Verification items for the finished model (mm, model axes). Round coordinates to 2 decimals unless told otherwise and drop trailing zeros. Write each loop counter-clockwise with the first axis right and the second up, starting at its lowest first coordinate (ties: lowest second). Pieces come first, ordered by that corner, then holes. Notation, with made-up numbers: (45, -3) -> (78, -3) arc R29 cw to (78, 36) -> close; hole circle Ø1 at (-6, 58). An arc over 180 degrees is marked (long way). Use CSV: the item, a comma, the result in double quotes.
```python
from build123d import *

# Parameters (mm, degrees)
BOSS_EXTRUDE1_DEPTH = 119.85625
SKETCH2_R           = 2.032
CUT_EXTRUDE1_DEPTH  = 136.095780221
SKETCH3_R           = 2.032
CUT_EXTRUDE2_DEPTH  = 12.7


with BuildPart() as part:
    # Sketch1 → Boss-Extrude1 (new, symmetric)
    with BuildSketch(Plane(origin=(0, 0, 0), x_dir=(0, 0, -1), z_dir=(1, 0, 0))):
        Polygon((0, 0), (0, 3.184811635), (40.762900177, -0.022300578), (58.304880654, -17.260912049), (56.079483543, -19.525472204), (39.361772519, -3.096875365), align=None)
    extrude(amount=BOSS_EXTRUDE1_DEPTH, both=True)

    # Sketch2 → Cut-Extrude1 (cut, through all)
    with BuildSketch(Plane(origin=(0, 3.165218593, -0.249030642), x_dir=(1, 0, 0), z_dir=(0, 0.9969192417821154, -0.0784348478966589))):
        with Locations(Location((113.50625, 6.354926815, 0), (0, 0, 270))):
            Circle(SKETCH2_R)
        with Locations(Location((-113.50625, 6.354926815, 0), (0, 0, 270))):
            Circle(SKETCH2_R)
    extrude(amount=-CUT_EXTRUDE1_DEPTH, mode=Mode.SUBTRACT)

    # Sketch3 → Cut-Extrude2 (cut)
    with BuildSketch(Plane(origin=(0, 20.36700431, -20.014779664), x_dir=(1, 0, 0), z_dir=(0, 0.7132472930974809, -0.7009124759120187))):
        with Locations(Location((-113.50625, 45.429186901, 0), (0, 0, 270))):
            Circle(SKETCH3_R)
        with Locations(Location((113.50625, 48.604186901, 0), (0, 0, 270))):
            Circle(SKETCH3_R)
    extrude(amount=-CUT_EXTRUDE2_DEPTH, mode=Mode.SUBTRACT)


solid = part.part
```
Q1. Mould release check, pull along X, two halves, no side actions. Record for faces 1 (the flat face through (-119.856, -2, -31)), 2 (the flat face through (1.68, -1.57, -19.96)), 3 (the cylindrical face through (-115.49, -12.9, -51.63)): released by +X, released by -X, zero draft, split by the parting line, or undercut.
Filled in:
face 1,"released by -X"
face 2,"zero draft"
face 3,"undercut"
Q2. Section check C-C (z = -33). Record the cut outline in (x, y), plus the area to 3 significant figures.
Filled in:
outline,"(-119.86, -2.6) -> (119.86, -2.6) -> (119.86, 0.59) -> (-119.86, 0.59) -> close"
area,"763 mm²"
Q3. Section check B-B (z = -46). Record the cut outline in (x, y).
Filled in:
outline,"(-119.86, -9.62) -> (119.86, -9.62) -> (119.86, -5.17) -> (-119.86, -5.17) -> close"
Q4. Material ranges on L1, parallel to Z at x = -99.5, y = -16.25; L2, parallel to Y at x = -81.5, z = -20.5; L3, parallel to Y at x = -22.5, z = -14.5, recorded low to high.
Filled in:
L1,"-57.28 to -52.75"
L2,"-1.61 to 1.57"
L3,"-1.14 to 2.04"
Q5. Go/stop test with flat-tipped pins: P1, Ø6, axis at x = 22, z = -9.5, coming from the +Y side; P2, Ø6, axis at x = 53.5, y = -17, coming from the -Z side; P3, Ø3, axis at x = -35, y = -7.5, coming from the -Z side; P4, Ø8, axis at x = 91, y = -11.5, coming from the -Z side. Record where each tip stops, or that it passes through.
Filled in:
P1,"y = 2.67"
P2,"z = -58.3"
P3,"z = -49.9"
P4,"z = -56.51"
Q6. Section check A-A (x = 104). Record the cut outline in (y, z).
Filled in:
outline,"(-19.53, -56.08) -> (-17.26, -58.3) -> (-0.02, -40.76) -> (3.18, 0) -> (0, 0) -> (-3.1, -39.36) -> close"
